```python
from build123d import *

# Parameters (mm, degrees)
SKETCH1_R               = 5
BOSS_EXTRUDE1_DEPTH     = 50
CUT_EXTRUDE1_DEPTH      = 52
CUT_EXTRUDE1_DEPTH_BACK = 35
SKETCH2_W               = 30
SKETCH2_H               = 60
SKETCH3_W               = 30
SKETCH3_H               = 40
CUT_EXTRUDE2_DEPTH      = 52
CUT_EXTRUDE3_START      = -10
CUT_EXTRUDE3_DEPTH      = 30
CUT_EXTRUDE4_START      = -10
CUT_EXTRUDE4_DEPTH      = 30
SKETCH6_R               = 25
BOSS_EXTRUDE2_DEPTH     = 30


with BuildPart() as part:
    # Sketch1 → Boss-Extrude1 (new body)
    with BuildSketch(Plane(origin=(0, 0, 0), x_dir=(0, 0, -1), z_dir=(1, 0, 0))):
        with BuildLine():
            Line((-255.87149894, 42.046001407), (44.12850106, 42.046001407))
            add(Edge.make_bspline(
                [(44.12850106, 42.046001407), (124.12850106, 17.046001407), (44.12850106, -7.953998593)],
                knots=[0, 0, 0, 1, 1, 1], degree=2))
            Line((44.12850106, -7.953998593), (-255.87149894, -7.953998593))
            add(Edge.make_bspline(
                [(-255.87149894, 42.046001407), (-335.87149894, 17.046001407), (-255.87149894, -7.953998593)],
                knots=[0, 0, 0, 1, 1, 1], degree=2))
        make_face()
        with Locations((-280.87149894, 17.046001407)):
            Circle(SKETCH1_R, mode=Mode.SUBTRACT)
        with Locations((69.12850106, 17.046001407)):
            Circle(SKETCH1_R, mode=Mode.SUBTRACT)
    extrude(amount=BOSS_EXTRUDE1_DEPTH)

    # Sketch2 → Cut-Extrude1 (cut, two sides: drawn at the far end of the back side and taken through both)
    with BuildSketch(Plane(origin=(0, 0, 0), x_dir=(1, 0, 0), z_dir=(0, 1, 0)).offset(-CUT_EXTRUDE1_DEPTH_BACK)):
        with Locations((25, 54.12850106)):
            Rectangle(SKETCH2_W, SKETCH2_H)
    extrude(amount=CUT_EXTRUDE1_DEPTH + CUT_EXTRUDE1_DEPTH_BACK, mode=Mode.SUBTRACT)

    # Sketch3 → Cut-Extrude2 (cut)
    with BuildSketch(Plane.XZ.offset(7.953998593)):
        with Locations((25, 275.87149894)):
            Rectangle(SKETCH3_W, SKETCH3_H)
    extrude(amount=-CUT_EXTRUDE2_DEPTH, mode=Mode.SUBTRACT)

    # Sketch4 → Cut-Extrude3 (cut)
    with BuildSketch(Plane.ZY.offset(CUT_EXTRUDE3_START)):
        Polygon((-24.12850106, 17.046001407), (-24.12850106, 42.046001407), (19.172769129, 42.046001407), align=None)
    extrude(amount=-CUT_EXTRUDE3_DEPTH, mode=Mode.SUBTRACT)

    # Sketch5 → Cut-Extrude4 (cut)
    with BuildSketch(Plane.ZY.offset(CUT_EXTRUDE4_START)):
        Polygon((-24.12850106, -7.953998593), (-24.12850106, 17.046001407), (19.172769129, -7.953998593), align=None)
    extrude(amount=-CUT_EXTRUDE4_DEPTH, mode=Mode.SUBTRACT)

    # Sketch6 → Boss-Extrude2 (add)
    with BuildSketch(Plane.XZ.offset(7.953998593)):
        with Locations(Location((25, 75.87149894, 0), (0, 0, 180))):
            Circle(SKETCH6_R)
    extrude(amount=BOSS_EXTRUDE2_DEPTH)


solid = part.part
```
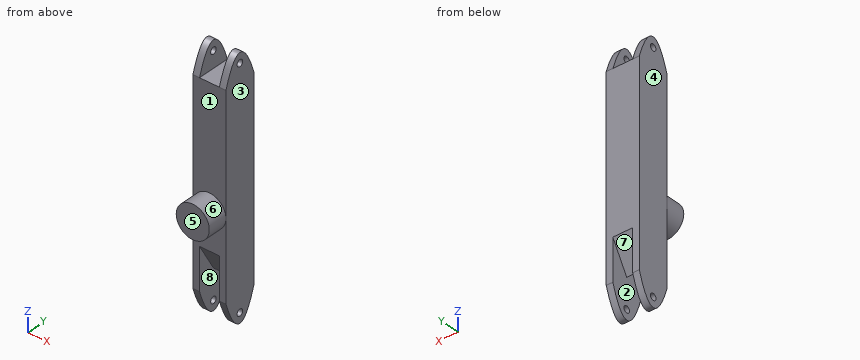
Verification items for the finished model (mm, model axes). Face numbers are marked on the shaded views. A direction names the side the tool comes from. Coordinates: 2 decimals unless noted, no trailing zeros. Loops run counter-clockwise (first coordinate to the right, second up) from the corner with the lowest first, then second, coordinate; pieces in that order, holes last. Notation, with made-up numbers: (0.5, 81.5) -> (27.5, 81.5) arc R13 ccw to (27.5, 87.5) -> close; hole circle Ø9 at (73.25, 26.25). An arc over 180 degrees is marked (long way). Answer in a Markdown table with one row per item.
1) Section check A-A (x = 25). Record the cut outline in (y, z), and give its area (3 significant figures).
The answers:
| item | result |
|---|---|
| outline | (-37.95, 50.87) -> (-7.95, 50.87) -> (-7.95, 19.17) -> (17.05, -24.13) -> (42.05, 19.17) -> (42.05, 255.87) -> (-7.95, 255.87) -> (-7.95, 100.87) -> (-37.95, 100.87) -> close |
| area | 14,400 mm2 |
2) Section check B-B (z = 233.5). Record the cut outline in (x, y).
The answers:
| item | result |
|---|---|
| outline | (0, -7.95) -> (50, -7.95) -> (50, 42.05) -> (0, 42.05) -> close |
3) Access from +Z, -Z, +X, -X, +Y, -Y to the whole of each face (thin tool, end or side, straight path). Record for the marked faces 4, 5, 6, 7 and 8.
The answers:
| item | result |
|---|---|
| face 4 | +Z, -Z, -X, +Y, -Y |
| face 5 | +Z, -Z, +X, -X, -Y |
| face 6 | -Y |
| face 7 | -Z, +Y |
| face 8 | -Z |
4) Draft check along X on the marked faces 1, 2 and 3. Enter one of: released by +X, released by -X, zero draft, split by the parting line, or undercut.
The answers:
| item | result |
|---|---|
| face 1 | zero draft |
| face 2 | undercut |
| face 3 | released by +X |
5) Scan lines: line 1 along Z through (x, y) = (2, 17.5); line 2 along X through (y, z) = (10.5, -52.5); line 3 along Y through (x, z) = (21.5, 247.5). Record each from-to range of solid material in increasing order. Write a range as from..to.
The answers:
| item | result |
|---|---|
| line 1 | z = -84.12..-74.11, -64.15..275.89, 285.85..295.86 |
| line 2 | x = 0..10, 40..50 |
| line 3 | y = -7.95..42.05 |
6) Depth check by flat-ended pin: P1, Ø8, axis at x = 40.5, y = -2.5, coming from the -Z side; P2, Ø15, axis at x = 29, z = 43, coming from the -Y side; P3, Ø1.5, axis at y = -27.5, z = 86, coming from the -X side. Enter the tip coordinate at first touch or a pass-through.
The answers:
| item | result |
|---|---|
| P1 | stops at z = -68.66 |
| P2 | stops at y = -7.95 |
| P3 | stops at x = 1.83 |
